```python
from build123d import *

# Parameters (mm, degrees)
SKETCH_1_W                = 36
SKETCH_1_H                = 10
BLOCKEXTRUDE_DEPTH        = 58
FILLET_2_R                = 2
SKETCH_2_R                = 6.3
DRIVE_SHAFT_PASSAGE_DEPTH = 69.992753243


with BuildPart() as part:
    # 草图1 → BlockExtrude (new body)
    with BuildSketch(Plane.XY):
        with Locations((18, 5)):
            Rectangle(SKETCH_1_W, SKETCH_1_H)
    extrude(amount=BLOCKEXTRUDE_DEPTH)

    # Fillet 2
    fillet_2_edges = [part.edges().sort_by_distance(p)[0] for p in [
        (36, 5, 58),
        (0, 5, 58),
        (36, 5, 0),
        (0, 5, 0),
    ]]
    fillet(fillet_2_edges, radius=FILLET_2_R)

    # 草图2 → Drive_shaft_passage (cut, through all)
    with BuildSketch(Plane(origin=(0, 10, 0), x_dir=(1, 0, 0), z_dir=(0, 1, 0))):
        with Locations(Location((18, -24.5744, 0), (0, 0, 270))):
            Circle(SKETCH_2_R)
    extrude(amount=-DRIVE_SHAFT_PASSAGE_DEPTH, mode=Mode.SUBTRACT)


solid = part.part
```
The listing builds one solid part. Answer for the finished solid, in the listing's coordinates (mm). Give positions to 0.01 mm unless a question says otherwise; leave off trailing zeros. Write each loop counter-clockwise with the first axis right and the second up, starting at its lowest first coordinate (ties: lowest second). Pieces come first, ordered by that corner, then holes. Notation, with made-up numbers: (75, -17) -> (90, -17) arc R31 ccw to (90, 12) -> close; hole circle Ø8 at (-22, -15.5). An arc over 180 degrees is marked (long way). Write item = value, one per line. Start each with the question number.
1) Determine the mould class of faces 1 (the face through (0.57, 5.07, 0.6)), 2 (the face through (22.258, 5.07, 19.931)), 3 (the face through (18, 0, 35)) for opening direction X: +X half, -X half, draft (parallel to the pull), parting line (faces both ways), or undercut.
2) The part is cut by section B-B, the plane y = 8.5. Determine the outline of the cut face in (x, z), and give its area (3 significant figures).
3) The part is cut by section A-A, the plane x = 18. Determine the outline of the cut face in (y, z), and give its area (3 significant figures).
4) The part is cut by section C-C, the plane z = 20. Determine the outline of the cut face in (x, y), and give its area (3 significant figures).
5) This flat-tipped pin is pushed along its axis until it touches: pin 1 (4 mm diameter, centred on x = 6.5, z = 17.5, fed in from -Y). Where does it stop, or does it pass through?
6) Straight lines are drawn through the part: line 1 along Z through (x, y) = (21.5, 5.75); line 2 along Z through (x, y) = (13, 4.5). For each, find the intervals that lie inside material, in ascending order.
Solutions:
q1.face_1 = -X half
q1.face_2 = undercut
q1.face_3 = draft
q2.outline = (0, 2) arc R2 ccw to (2, 0) -> (34, 0) arc R2 ccw to (36, 2) -> (36, 56) arc R2 ccw to (34, 58) -> (2, 58) arc R2 ccw to (0, 56) -> close; hole circle Ø12.6 at (18, 24.57)
q2.area = 1,960 mm²
q3.outline = (0, 0) -> (10, 0) -> (10, 18.27) -> (0, 18.27) -> close; (0, 30.87) -> (10, 30.87) -> (10, 58) -> (0, 58) -> close
q3.area = 454 mm²
q4.outline = (0, 0) -> (13.67, 0) -> (13.67, 10) -> (0, 10) -> close; (22.33, 0) -> (36, 0) -> (36, 10) -> (22.33, 10) -> close
q4.area = 273 mm²
q5.pin_1 = 0
q6.line_1 = 0 to 19.34, 29.81 to 58
q6.line_2 = 0 to 20.74, 28.41 to 58
